Can you work these out from the drawing? Everything is in mm from the part's minimum corner. A direction names the side the tool comes from. Give positions to 0.01 mm unless a question says otherwise; leave off trailing zeros. Loops run counter-clockwise (first coordinate to the right, second up) from the corner with the lowest first, then second, coordinate; pieces in that order, holes last.
Q1. If we section it at D-D (z = 38.5): Please give me the cut outline in (x, y) (1 decimal).
Q2. If we section it at C-C (y = 21.25): Please give me the cut outline in (x, z), plus the area to 3 significant figures.
Q3. If we section it at A-A (z = 6): Please give me the cut outline in (x, y).
Q4. Will these pins go through, and if not, where does the flat tip stop? P1, Ø7, axis at y = 19, z = 28, coming from the -X side; P2, Ø8, axis at x = 14, z = 75, coming from the +Y side; P3, Ø12, axis at x = 15, y = 15.5, coming from the -Z side.
Q5. For the marked faces 1 and 2, which set-ups out of +Z, -Z, +X, -X, +Y, -Y let a thin tool reach every point of the face, with its end or its side?
Q6. I need wall thicknesses on line 1 (X direction, y = 5.5, z = 18); line 2 (Y direction, x = 12.5, z = 37.5); line 3 (Z direction, x = 24.25, y = 16.5). Which ranges of each line are inside material? Lowest first, please.
Q7. If we section it at B-B (x = 19): Please give me the cut outline in (y, z), plus the area to 3 significant figures.
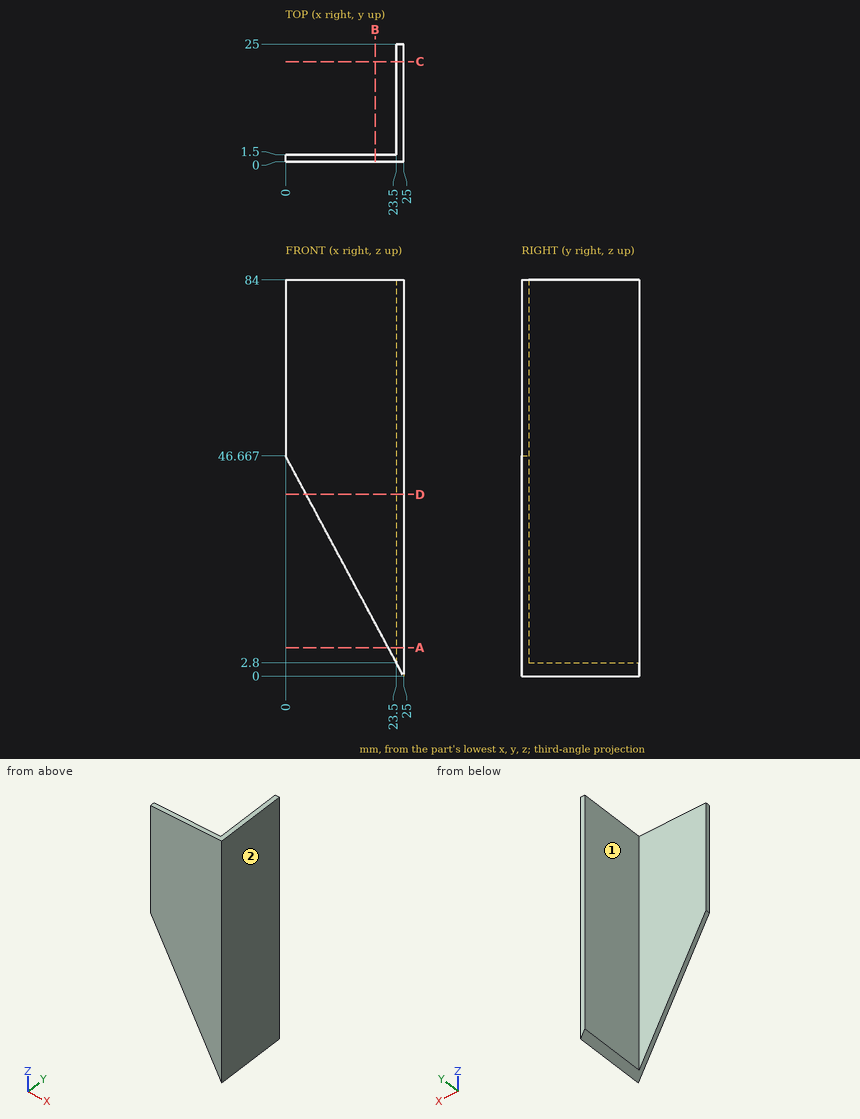
Check sheet entries:
1. outline: (4.4, 0) - (25, 0) - (25, 25) - (23.5, 25) - (23.5, 1.5) - (4.4, 1.5) - close
2. outline: (23.5, 2.8) - (25, 0) - (25, 84) - (23.5, 84) - close
2. area: 124 mm2
3. outline: (21.79, 0) - (25, 0) - (25, 25) - (23.5, 25) - (23.5, 1.5) - (21.79, 1.5) - close
4. P1: stops at x = 23.5
4. P2: stops at y = 1.5
4. P3: passes through
5. face 1: +Z, -Z, -X, +Y
5. face 2: +Z, -Z, +X, +Y, -Y
6. line 1: x = 23.5 to 25
6. line 2: y = 0 to 1.5
6. line 3: z = 1.4 to 84
7. outline: (0, 11.2) - (1.5, 11.2) - (1.5, 84) - (0, 84) - close
7. area: 109 mm2
